Build history of the part. All positions in model axes, mm. A direction names the side the tool comes from. Round coordinates to 2 decimals unless told otherwise and drop trailing zeros. Loops run counter-clockwise (first coordinate to the right, second up) from the corner with the lowest first, then second, coordinate; pieces in that order, holes last. Notation, with made-up numbers: M 23.5,36.25 L 80.5,36.25 A21 ccw 80.5,41.25 Z; hole C -22.75,64.5 d9. An arc over 180 degrees is marked long. One line per item, written item: value.
```python
from build123d import *

# Parameters (mm, degrees)
SKETCH1_R           = 12.485
BOSS_EXTRUDE1_DEPTH = 20
SKETCH2_R           = 15
BOSS_EXTRUDE2_DEPTH = 15
SKETCH3_R           = 4.5
BOSS_EXTRUDE3_DEPTH = 55
SKETCH4_R           = 4.8
BOSS_EXTRUDE4_DEPTH = 5
BOSS_EXTRUDE4_DRAFT = -20
SKETCH5_R           = 6.619851171
BOSS_EXTRUDE6_DEPTH = 5
FILLET1_R           = 5
FILLET2_R           = 5
CUT_EXTRUDE2_START  = -15
SKETCH6_R           = 12.485
CUT_EXTRUDE2_DEPTH  = 15


# Some blends are built 0.0001 mm under size
with BuildPart() as part:
    # Sketch1 → Boss-Extrude1 (new body)
    with BuildSketch(Plane.XY):
        Circle(SKETCH1_R)
    extrude(amount=BOSS_EXTRUDE1_DEPTH)

    # Sketch2 → Boss-Extrude2 (add)
    with BuildSketch(Plane(origin=(0, 0, 0), x_dir=(-1, 0, 0), z_dir=(0, 0, -1))):
        Circle(SKETCH2_R)
    extrude(amount=BOSS_EXTRUDE2_DEPTH)

    # Sketch3 → Boss-Extrude3 (add)
    with BuildSketch(Plane(origin=(0, 0, 0), x_dir=(0, 0, -1), z_dir=(1, 0, 0))):
        with Locations((7.5, 0)):
            Circle(SKETCH3_R)
    extrude(amount=BOSS_EXTRUDE3_DEPTH)


with BuildPart() as boss_extrude4_tool:
    # Sketch4 → Boss-Extrude4 (with draft: the straight prism first)
    with BuildSketch(Plane(origin=(55, 0, 0), x_dir=(0, 0, -1), z_dir=(1, 0, 0))):
        with Locations((7.5, 0)):
            Circle(SKETCH4_R)
    extrude(amount=BOSS_EXTRUDE4_DEPTH)
    # Boss-Extrude4: the draft: its side faces are tilted about the plane it starts from
    boss_extrude4_sides = [boss_extrude4_tool.faces().sort_by_distance(p)[0] for p in [
        (57.5, 0, -2.7),
    ]]
    draft(boss_extrude4_sides, Plane(origin=(55, 0, 0), x_dir=(0, 0, -1), z_dir=(1, 0, 0)), BOSS_EXTRUDE4_DRAFT)


with BuildPart() as part_1:
    add(part.part)

    # Boss-Extrude4: add boss_extrude4_tool
    add(boss_extrude4_tool.part)

    # Sketch5 → Boss-Extrude6 (add)
    with BuildSketch(Plane(origin=(60, 0, 0), x_dir=(0, 0, -1), z_dir=(1, 0, 0))):
        with Locations((7.5, 0)):
            Circle(SKETCH5_R)
    extrude(amount=BOSS_EXTRUDE6_DEPTH)

    # Fillet1
    fillet1_edges = [part_1.edges().sort_by_distance(p)[0] for p in [
        (65, 0, -0.880148829),
    ]]
    fillet(fillet1_edges, radius=FILLET1_R - 0.0001)  # a hair under: the kernel refuses the full size

    # Fillet2
    # the kernel refuses this fillet: 5 mm, written as the material it adds along each edge
    with BuildSketch(Plane(origin=(55, 0, -7.5), x_dir=(0, 0, -1), z_dir=(0, -1, 0))) as fillet2_piece_1:
        with BuildLine():
            CenterArc((9.5, -1.705872211), FILLET2_R, 160.051556411, 19.948443589)
            Line((4.5, -1.705872211), (4.4, -1.705872211))
            Line((4.4, -1.705872211), (4.4, 0))
            Line((4.4, 0), (4.5, 0.1))
            ThreePointArc((4.5, 0.1), (4.65, 0.1), (4.706, 0.034117444))
            Line((4.706, 0.034117444), (4.8, 0))
        make_face()
    revolve(axis=Axis((55, 0, -7.5), (1, 0, 0)))

    # Sketch6 → Cut-Extrude2 (cut)
    with BuildSketch(Plane.XY.offset(20).offset(CUT_EXTRUDE2_START)):
        Circle(SKETCH6_R)
    extrude(amount=CUT_EXTRUDE2_DEPTH, mode=Mode.SUBTRACT)


solid = part_1.part
```
Item 1: Wall check: line 1 along Z through (x, y) = (-9, 10); line 2 along X through (y, z) = (-11, -12.25); line 3 along Y through (x, z) = (38.5, -7). Give the ranges that are in metal, low to high.
Check values:
line 1: z = -15 to 0
line 2: x = -10.2 to 10.2
line 3: y = -4.47 to 4.47
Item 2: Drop flat-ended pins along their axis: P1, Ø10, axis at x = 45, z = -4.5, coming from the +Y side; P2, Ø1.5, axis at x = -6.5, z = -12.5, coming from the +Y side; P3, Ø6, axis at x = 57, z = -4.5, coming from the +Y side. Give the stop position or say it passes through.
Check values:
P1: stops at y = 4.5
P2: stops at y = 13.85
P3: stops at y = 6.3
Item 3: Which spindle directions (+Z, -Z, +X, -X, +Y, -Y) get a long thin tool onto all of the face, cutting with end or side? Do faces 1 (the face through (0, 0, 5)), 2 (the face through (3.4, 12.3, 0)). Say none if no direction does.
Check values:
face 1: +Z, +X, -X, +Y, -Y
face 2: +Z
Item 4: Slice it at A-A, the plane x = 0. Give the cut face in (y, z) (3 decimals).
Check values:
outline: M -15,-15 L 15,-15 L 15,0 L 12.485,0 L 12.485,5 L -12.485,5 L -12.485,0 L -15,0 Z
Item 5: Pull direction X, two halves, no side cores. Call faces 3 (the face through (0, 0, -15)), 4 (the face through (55.798, 1.529, -12.355)), 5 (the face through (33.529, 1.352, -11.792)), 6 (the face through (-1.63, 12.38, 2.46)): pulls with the +X half, pulls with the -X half, needs draft (parallel to the pull), parting line crosses it, or undercut.
Check values:
face 3: needs draft
face 4: undercut
face 5: undercut
face 6: parting line crosses it
Item 6: Slice it at D-D, the plane x = 50. Give the cut face in (y, z).
Check values:
outline: C 0,-7.5 d9
Item 7: Slice it at B-B, the plane z = 2.25. Give the cut face in (x, y) (3 decimals), and give its area (3 significant figures).
Check values:
outline: C 0,0 d24.97
area: 490 mm2
Item 8: Slice it at C-C, the plane y = -11.5. Give the cut face in (x, z).
Check values:
outline: M -9.63,-15 L 9.63,-15 L 9.63,0 L 4.86,0 L 4.86,5 L -4.86,5 L -4.86,0 L -9.63,0 Z
